```python
from build123d import *

# Parameters (mm, degrees)
SKETCH1_R           = 1.3
SKETCH1_W           = 3
SKETCH1_H           = 10
BOSS_EXTRUDE2_DEPTH = 3
SKETCH1_5_W         = 3
SKETCH1_5_H         = 10
BOSS_EXTRUDE3_DEPTH = 23.85
SKETCH4_R           = 1.575411087
CUT_EXTRUDE1_DEPTH  = 3


with BuildPart() as part:
    # Sketch1 → Boss-Extrude2 (new body)
    # profile 1 of 2: a face of its own
    with BuildSketch(Plane(origin=(0, 0, 0), x_dir=(1, 0, 0), z_dir=(0, 1, 0))):
        Polygon((-14.75, 16), (-14.75, 10.5), (9.25, 10.5), (9.25, -10.5), (-14.75, -10.5), (-14.75, -16), (14.75, -16), (14.75, -5), (30.2, -5), (30.2, 5), (14.75, 5), (14.75, 16), align=None)
        with Locations(Location((-11.5, -13.5, 0), (0, 0, 270))):
            Circle(SKETCH1_R, mode=Mode.SUBTRACT)
        with Locations(Location((-3.5, -13.5, 0), (0, 0, 270))):
            Circle(SKETCH1_R, mode=Mode.SUBTRACT)
        with Locations(Location((-11.5, 13.5, 0), (0, 0, 270))):
            Circle(SKETCH1_R, mode=Mode.SUBTRACT)
        with Locations(Location((-3.5, 13.5, 0), (0, 0, 270))):
            Circle(SKETCH1_R, mode=Mode.SUBTRACT)
    # profile 2 of 2: a face of its own
    with BuildSketch(Plane(origin=(0, 0, 0), x_dir=(1, 0, 0), z_dir=(0, 1, 0))):
        with Locations((31.7, 0)):
            Rectangle(SKETCH1_W, SKETCH1_H)
    extrude(amount=-BOSS_EXTRUDE2_DEPTH)

    # Sketch1<5> → Boss-Extrude3 (add)
    with BuildSketch(Plane(origin=(0, 0, 0), x_dir=(1, 0, 0), z_dir=(0, 1, 0))):
        with Locations((31.7, 0)):
            Rectangle(SKETCH1_5_W, SKETCH1_5_H)
    extrude(amount=-BOSS_EXTRUDE3_DEPTH)

    # Sketch4 → Cut-Extrude1 (cut)
    with BuildSketch(Plane.ZY.offset(-30.2)):
        with Locations((0, -18.85)):
            Circle(SKETCH4_R)
    extrude(amount=-CUT_EXTRUDE1_DEPTH, mode=Mode.SUBTRACT)


solid = part.part
```
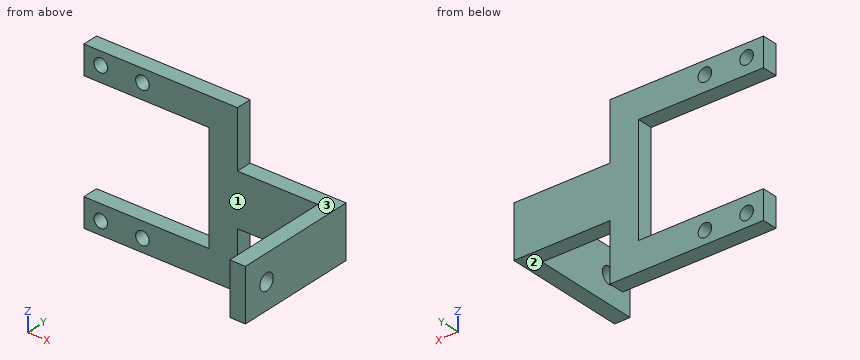
Model file for the job. Use its own axes, mm. Face numbers are marked on the shaded views. A direction names the side the tool comes from. Give positions to 0.01 mm unless a question says otherwise; leave off trailing zeros. Order: outer loops, then holes, each group sorted by start corner. A loop starts at its lowest first (then second) coordinate and runs counter-clockwise, first axis right, second up.
1) Wall check: probe 1 along X at (y, z) = (-2.35, -13.5); probe 2 along X at (y, z) = (-9, 3); probe 3 along Y at (x, z) = (10.5, 7.5). Give the ranges that are in metal, low to high.
2) 3-axis set-ups, long thin cutter, end or side, ignore diameter. For the marked faces 1, 2 and 3: which of +Z, -Z, +X, -X, +Y, -Y reach the whole face in a straight line?
3) Saw through at A-A, the plane z = 13.5. Write the cut outline in (x, y).
4) Saw through at C-C, the plane z = 0. Write the cut outline in (x, y).
5) Pin check, flat tips, straight feed: pin 1 (8 mm diameter, centred on y = -12, z = -2, fed in from -X); pin 2 (3 mm diameter, centred on y = -18.85, z = 0, fed in from +X); pin 3 (8 mm diameter, centred on x = 13, z = 7.5, fed in from +Y); pin 4 (0.9 mm diameter, centred on y = -1.5, z = -13, fed in from +X). Stop position of each tip, or through.
6) Saw through at B-B, the plane x = -11.5. Write the cut outline in (y, z), then the cut area to 3 significant figures.
7) Saw through at D-D, the plane x = 6. Write the cut outline in (y, z).
Computed:
1. probe 1: x = -14.75 to -12.8, -10.2 to -4.8, -2.2 to 14.75
1. probe 2: x = 30.2 to 33.2
1. probe 3: y = -3 to 0
2. face 1: +Z, -Z, -X, -Y
2. face 2: -Z, +X, +Y, -Y
2. face 3: +Z, +X, +Y, -Y
3. outline: (-14.75, -3) - (-12.8, -3) - (-12.8, 0) - (-14.75, 0) - close; (-10.2, -3) - (-4.8, -3) - (-4.8, 0) - (-10.2, 0) - close; (-2.2, -3) - (14.75, -3) - (14.75, 0) - (-2.2, 0) - close
4. outline: (9.25, -3) - (30.2, -3) - (30.2, -17.27) - (33.2, -17.27) - (33.2, 0) - (9.25, 0) - close; (30.2, -23.85) - (33.2, -23.85) - (33.2, -20.43) - (30.2, -20.43) - close
5. pin 1: stops at x = 30.2
5. pin 2: passes through
5. pin 3: stops at y = 0
5. pin 4: stops at x = 14.75
6. outline: (-3, -16) - (0, -16) - (0, -14.8) - (-3, -14.8) - close; (-3, -12.2) - (0, -12.2) - (0, -10.5) - (-3, -10.5) - close; (-3, 10.5) - (0, 10.5) - (0, 12.2) - (-3, 12.2) - close; (-3, 14.8) - (0, 14.8) - (0, 16) - (-3, 16) - close
6. area: 17.4 mm2
7. outline: (-3, -16) - (0, -16) - (0, -10.5) - (-3, -10.5) - close; (-3, 10.5) - (0, 10.5) - (0, 16) - (-3, 16) - close
